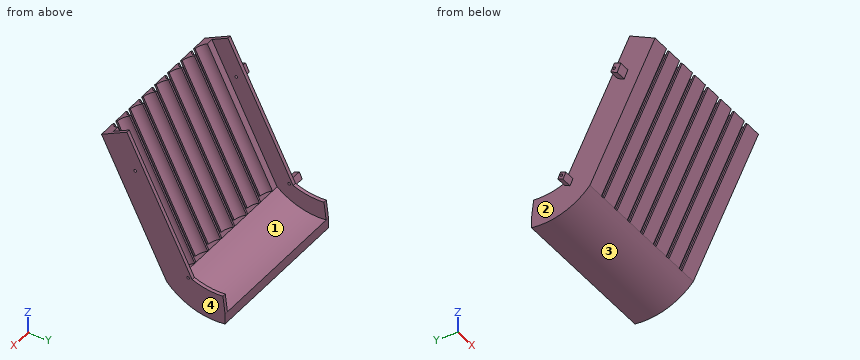
```python
from build123d import *

# Parameters (mm, degrees)
BOSS_EXTRUDE1_DEPTH      = 1234.900343145
BOSS_EXTRUDE1_DEPTH_BACK = 82.174065831
CUT_EXTRUDE1_DEPTH       = 1200
BOSS_EXTRUDE2_DEPTH      = 30
BOSS_EXTRUDE3_DEPTH      = 30
BOSS_EXTRUDE4_START      = -30
BOSS_EXTRUDE4_DEPTH      = 30
BOSS_EXTRUDE5_DEPTH      = 30
BOSS_EXTRUDE6_DEPTH      = 90
CUT_EXTRUDE2_DEPTH       = 1710
CUT_EXTRUDE2_DEPTH_BACK  = 1710
SKETCH12_R               = 11.090448241
SKETCH12_R_2             = 10.749574141


with BuildPart() as part:
    # Sketch1 → Boss-Extrude1 (new, two sides: drawn at the far end of the back side and taken through both)
    with BuildSketch(Plane(origin=(0, 0, 0), x_dir=(0, 0, -1), z_dir=(1, 0, 0)).offset(-BOSS_EXTRUDE1_DEPTH_BACK)):
        Polygon((1029.256665049, 623.197173816), (1069.207829026, 544.788599687), (0, 0), (-39.951163977, 78.408574129), align=None)
        with BuildLine():
            Line((1029.256665049, 623.197173816), (1069.207829026, 544.788599687))
            ThreePointArc((1069.207829026, 544.788599687), (1215.235027559, 767.659323729), (1237.256665049, 1033.197173816))
            Line((1237.256665049, 1033.197173816), (1149.256665049, 1033.197173816))
            ThreePointArc((1149.256665049, 1033.197173816), (1131.408548141, 815.860037301), (1029.256665049, 623.197173816))
        make_face()
    extrude(amount=BOSS_EXTRUDE1_DEPTH + BOSS_EXTRUDE1_DEPTH_BACK)

    # Sketch2 → Cut-Extrude1 (cut)
    with BuildSketch(Plane(origin=(0, 0, 0), x_dir=(1, 0, 0), z_dir=(0, -0.45399049973954786, 0.8910065241883673))):
        with BuildLine():
            ThreePointArc((98.567789191, 15), (140.165131778, 41.445455593), (156.363138657, 88))
            Line((156.363138657, 88), (6.363138657, 88))
            ThreePointArc((6.363138657, 88), (22.561145536, 41.445455593), (64.158488123, 15))
            Line((64.158488123, 15), (64.158488123, 0))
            Line((64.158488123, 0), (98.567789191, 0))
            Line((98.567789191, 0), (98.567789191, 15))
        make_face()
        with BuildLine():
            ThreePointArc((263.567789191, 15), (305.165131778, 41.445455593), (321.363138657, 88))
            Line((321.363138657, 88), (171.363138657, 88))
            ThreePointArc((171.363138657, 88), (187.561145536, 41.445455593), (229.158488123, 15))
            Line((229.158488123, 15), (229.158488123, 0))
            Line((229.158488123, 0), (263.567789191, 0))
            Line((263.567789191, 0), (263.567789191, 15))
        make_face()
        with BuildLine():
            ThreePointArc((428.567789191, 15), (470.165131778, 41.445455593), (486.363138657, 88))
            Line((486.363138657, 88), (336.363138657, 88))
            ThreePointArc((336.363138657, 88), (352.561145536, 41.445455593), (394.158488123, 15))
            Line((394.158488123, 15), (394.158488123, 0))
            Line((394.158488123, 0), (428.567789191, 0))
            Line((428.567789191, 0), (428.567789191, 15))
        make_face()
        with BuildLine():
            Line((651.363138657, 88), (501.363138657, 88))
            ThreePointArc((501.363138657, 88), (517.561145536, 41.445455593), (559.158488123, 15))
            Line((559.158488123, 15), (559.158488123, 0))
            Line((559.158488123, 0), (593.567789191, 0))
            Line((593.567789191, 0), (593.567789191, 15))
            ThreePointArc((593.567789191, 15), (635.165131778, 41.445455593), (651.363138657, 88))
        make_face()
        with BuildLine():
            Line((816.363138657, 88), (666.363138657, 88))
            ThreePointArc((666.363138657, 88), (682.561145536, 41.445455593), (724.158488123, 15))
            Line((724.158488123, 15), (724.158488123, 0))
            Line((724.158488123, 0), (758.567789191, 0))
            Line((758.567789191, 0), (758.567789191, 15))
            ThreePointArc((758.567789191, 15), (800.165131778, 41.445455593), (816.363138657, 88))
        make_face()
        with BuildLine():
            Line((981.363138657, 88), (831.363138657, 88))
            ThreePointArc((831.363138657, 88), (847.561145536, 41.445455593), (889.158488123, 15))
            Line((889.158488123, 15), (889.158488123, 0))
            Line((889.158488123, 0), (923.567789191, 0))
            Line((923.567789191, 0), (923.567789191, 15))
            ThreePointArc((923.567789191, 15), (965.165131778, 41.445455593), (981.363138657, 88))
        make_face()
        with BuildLine():
            Line((1146.363138657, 88), (996.363138657, 88))
            ThreePointArc((996.363138657, 88), (1012.561145536, 41.445455593), (1054.158488123, 15))
            Line((1054.158488123, 15), (1054.158488123, 0))
            Line((1054.158488123, 0), (1088.567789191, 0))
            Line((1088.567789191, 0), (1088.567789191, 15))
            ThreePointArc((1088.567789191, 15), (1130.165131778, 41.445455593), (1146.363138657, 88))
        make_face()
    extrude(amount=-CUT_EXTRUDE1_DEPTH, mode=Mode.SUBTRACT)

    # Sketch3 → Boss-Extrude2 (add)
    with BuildSketch(Plane(origin=(1234.900343145, 0, 0), x_dir=(0, 0, -1), z_dir=(1, 0, 0))):
        Polygon((-39.951163977, 78.408574129), (-108.049738938, 212.059552757), (961.158090088, 756.848152444), (1029.256665049, 623.197173816), align=None)
    extrude(amount=-BOSS_EXTRUDE2_DEPTH)

    # Sketch6 → Boss-Extrude3 (add)
    with BuildSketch(Plane.ZY.offset(82.174065831)):
        Polygon((-1029.256665049, 623.197173816), (-961.158090088, 756.848152444), (108.049738938, 212.059552757), (39.951163977, 78.408574129), align=None)
    extrude(amount=-BOSS_EXTRUDE3_DEPTH)

    # Sketch9 → Boss-Extrude4 (add)
    with BuildSketch(Plane(origin=(1234.900343145, 0, 0), x_dir=(0, 0, -1), z_dir=(1, 0, 0)).offset(BOSS_EXTRUDE4_START)):
        with BuildLine():
            Line((1149.256665049, 1033.197173816), (1000.350769421, 1015.113085582))
            ThreePointArc((1000.350769421, 1015.113085582), (996.565266489, 883.581264805), (961.158090088, 756.848152444))
            Line((961.158090088, 756.848152444), (1029.256665049, 623.197173816))
            ThreePointArc((1029.256665049, 623.197173816), (1131.408548141, 815.860037301), (1149.256665049, 1033.197173816))
        make_face()
    extrude(amount=BOSS_EXTRUDE4_DEPTH)

    # Sketch10 → Boss-Extrude5 (add)
    with BuildSketch(Plane.ZY.offset(82.174065831)):
        with BuildLine():
            Line((-1029.256665049, 623.197173816), (-961.158090088, 756.848152444))
            ThreePointArc((-961.158090088, 756.848152444), (-996.565266489, 883.581264805), (-1000.350769421, 1015.113085582))
            Line((-1000.350769421, 1015.113085582), (-1149.256665049, 1033.197173816))
            ThreePointArc((-1149.256665049, 1033.197173816), (-1131.408548141, 815.860037301), (-1029.256665049, 623.197173816))
        make_face()
    extrude(amount=-BOSS_EXTRUDE5_DEPTH)

    # Sketch11 → Boss-Extrude6 (add)
    with BuildSketch(Plane.ZY.offset(82.174065831)):
        Polygon((-982.226090398, 754.490949456), (-929.767856808, 729.642312493), (-950.23144019, 686.441414242), (-1002.68967378, 711.290051206), align=None)
        Polygon((-226.133327046, 312.103551466), (-158.807904246, 280.212561719), (-183.700784796, 227.660925002), (-251.919927814, 257.665172066), align=None)
    extrude(amount=BOSS_EXTRUDE6_DEPTH)

    # Sketch12 → Cut-Extrude2 (cut, two sides: drawn at the far end of the back side and taken through both)
    with BuildSketch(Plane(origin=(1234.900343145, 0, 0), x_dir=(0, 0, -1), z_dir=(1, 0, 0)).offset(-CUT_EXTRUDE2_DEPTH_BACK)):
        with Locations((204.62902054, 281.838763818)):
            Circle(SKETCH12_R)
        with Locations((961.389588636, 723.712275526)):
            Circle(SKETCH12_R_2)
    extrude(amount=CUT_EXTRUDE2_DEPTH + CUT_EXTRUDE2_DEPTH_BACK, mode=Mode.SUBTRACT)


solid = part.part
```
Verification items for the finished model (mm, model axes). Face numbers are marked on the shaded views. Coordinates: 2 decimals unless noted, no trailing zeros. Loops run counter-clockwise (first coordinate to the right, second up) from the corner with the lowest first, then second, coordinate; pieces in that order, holes last. Notation, with made-up numbers: (-28.75, 76.25) - (-20.75, 76.25) arc R14 ccw to (-20.75, 99.25) - close; hole circle Ø3 at (81, -24.5). An arc over 180 degrees is marked (long way). Return JSON: item names as keys, results as strings.
1. Section check A-A, the plane z = -786. Count the separate pieces of the cut face and the enclosed holes in it, then the cut area to 3 significant figures.
Established:
{"separate pieces": "8", "enclosed holes": "0", "area": "67,100 mm2"}
2. Thickness scan on L1, parallel to X at y = 548.5, z = -873.5; L2, parallel to Y at x = 312.5, z = -324; L3, parallel to Z at x = 356, y = 462. Record the ranges inside material, lowest first.
Established:
{"L1": "x = -82.17 to -52.17, 1204.9 to 1234.9", "L2": "y = 165.09 to 224.16", "L3": "z = -906.73 to -824.34"}
3. Mould release check, pull along X, two halves, no side actions. Record for the marked faces 1, 2, 3 and 4: +X half, -X half, draft (parallel to the pull), parting line (faces both ways), or undercut.
Established:
{"face 1": "undercut", "face 2": "-X half", "face 3": "draft", "face 4": "+X half"}
4. Section check B-B, the plane x = 193.5. Record the boundary of the cut face in (y, z), then the cut area to 3 significant figures.
Established:
{"outline": "(0, 0) - (544.79, -1069.21) arc R541.37 ccw to (1033.2, -1237.26) - (1033.2, -1149.26) arc R541.37 cw to (623.2, -1029.26) - (575.79, -1053.41) - (31, 15.8) - close", "area": "86,400 mm2"}
5. Go/stop test with flat-tipped pins: pin 1 (4 mm diameter, centred on x = 625, z = -491, fed in from -Y); pin 2 (13.5 mm diameter, centred on y = 281.84, z = -204.63, fed in from +X); pin 3 (6 mm diameter, centred on x = 927, y = 662, fed in from +Z); pin 4 (3 mm diameter, centred on x = 890, y = 721, fed in from -Z). Record where each tip stops, or that it passes through.
Established:
{"pin 1": "stops at y = 249.16", "pin 2": "passes through", "pin 3": "stops at z = -1056.41", "pin 4": "stops at z = -1197.39"}
